For this review, take the finished solid that the model builds, in its own axes (mm). Round coordinates to 2 decimals unless told otherwise and drop trailing zeros. Order: outer loops, then holes, each group sorted by start corner. A loop starts at its lowest first (then second) coordinate and runs counter-clockwise, first axis right, second up. Notation, with made-up numbers: (8.5, -23.5) -> (60.5, -23.5) arc R26 cw to (60.5, 15.5) -> close; hole circle Ø10 at (87, 75). An arc over 180 degrees is marked (long way). Use a Markdown table: item, result. Add a question column.
1) Consider section B-B (z = -0.9). State the section outline as (x, y) points.
2) Clearance check with flat-ended pins moving along their axes: P1, Ø2, axis at x = 29.79, y = 9, coming from the -Z side; P2, Ø5.5, axis at x = 69.59, y = 23, coming from the -Z side; P3, Ø4.5, axis at x = 69.59, y = 11, coming from the -Z side. State where each tip first meets the part, or that it passes through.
3) Consider section D-D (x = 81.5). State the section outline as (y, z) points.
4) Consider section A-A (y = 28.5). State the section outline as (x, z) points, plus the area to 3 significant figures.
5) Consider section C-C (y = 16.5). State the section outline as (x, z) points, plus the area to 3 significant figures.
6) Wall thickness on line 1 along X through (y, z) = (17.75, -0.5); line 2 along X through (y, z) = (23.5, -1); line 3 along X through (y, z) = (29.5, -1.1): over which ranges is each line inside the solid? List them lowest first. Write a range as [from, to].
Autodesk Inventor part; units mm, degrees
ref_plane "YZ Plane" through (0, 0, 0) normal (1, 0, 0) x (0, 1, 0)
ref_plane "XZ Plane" through (0, 0, 0) normal (0, 1, 0) x (-1, 0, 0)
ref_plane "XY Plane" through (0, 0, 0) normal (0, 0, 1) x (1, 0, 0)
sketch "Szkic1" plane through (0, 0, 0) normal (1, 0, 0) x (0, 1, 0)
  line L0 (6, 0) -> (6, -2)
  line L1 (6, -2) -> (33, -2)
  line L2 (33, -2) -> (33, 0)
  line L3 (33, 0) -> (6, 0)
  line L4 (31, 0) -> (31, 2.3) construction
  line L5 (6, 0) -> (31, 0) construction
  line L6 (6, 5) -> (6, 0) construction
  dimension "d1" = 2
  dimension "d27" = 2
extrude "Wyciągnięcie proste1" add sketch "Szkic1" along normal blind 98
sketch "Szkic2" plane through (0, 6, -2) normal (0, 0, -1) x (-1, 0, 0)
  circle A0 centre (-69.5896, 17) radius 1.2295 construction
  circle A1 centre (-69.5896, 5) radius 1.2295 construction
  circle A2 centre (-29.7896, 3) radius 1.2295 construction
hole "Otwór1" at (69.5896, 23, -2) at (69.5896, 11, -2) at (29.7896, 9, -2) direction (0, 0, 1) diameter 3.4 depth 5.5 tip angle 118 countersink diameter 6.9 countersink angle 84.225
sketch "Szkic3" plane through (0, 6, -2) normal (0, 0, -1) x (-1, 0, 0)
  line L0 (-32.2896, 0) -> (-32.2896, 25)
  line L1 (-27.0896, 4.55) -> (-24.3896, 4.55)
  line L2 (-24.3896, 4.55) -> (-24.3896, 14.55)
  line L3 (-24.3896, 14.55) -> (-27.0896, 14.55)
  line L4 (-27.0896, 14.55) -> (-27.0896, 4.55)
  line L5 (-30.2896, 23.9) -> (-27.2896, 23.9)
  line L6 (-27.2896, 23.9) -> (-27.2896, 17.2)
  line L7 (-27.2896, 17.2) -> (-30.2896, 17.2)
  line L8 (-30.2896, 17.2) -> (-30.2896, 23.9)
  point P0 (0, -6)
  dimension "d17" = 5.2
  dimension "d18" = 4.55
  dimension "d19" = 2.7
  dimension "d20" = 10
  dimension "d21" = 2
  dimension "d22" = 17.2
  dimension "d23" = 6.7
  dimension "d24" = 3
extrude "Wyciągnięcie proste2" cut sketch "Szkic3" against normal up to next
sketch "Sketch4" plane through (0, 0, 0) normal (-1, 0, 0) x (0, 0, 1)
  line L0 (-2, 6) -> (-2, 33) construction
  line L1 (-2, 6) -> (-2, 7.1547)
  line L2 (0, 6) -> (-2, 6)
  line L3 (-2, 7.1547) -> (0, 6)
  point P0 (0, 0)
  dimension "d31" = 30
extrude "Extrusion3" cut sketch "Sketch4" against normal through all
properties part number "Tyl" material "Aluminium 6061"
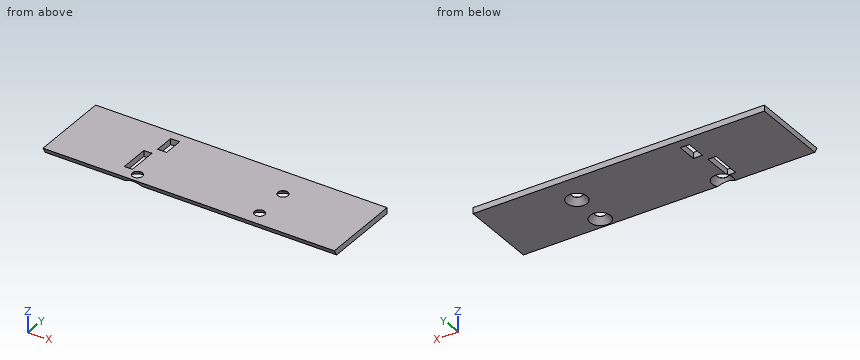
Results list:
| question | item | result |
|---|---|---|
| 1 | outline | (0, 6.52) -> (98, 6.52) -> (98, 33) -> (0, 33) -> close; hole (24.39, 10.55) -> (27.09, 10.55) -> (27.09, 20.55) -> (24.39, 20.55) -> close; hole (27.29, 23.2) -> (30.29, 23.2) -> (30.29, 29.9) -> (27.29, 29.9) -> close; hole circle Ø4.91 at (29.79, 9); hole circle Ø4.91 at (69.59, 11); hole circle Ø4.91 at (69.59, 23) |
| 2 | P1 | through |
| 2 | P2 | z = -1.23 |
| 2 | P3 | z = -0.67 |
| 3 | outline | (6, 0) -> (7.15, -2) -> (33, -2) -> (33, 0) -> close |
| 4 | outline | (0, -2) -> (27.29, -2) -> (27.29, 0) -> (0, 0) -> close; (30.29, -2) -> (98, -2) -> (98, 0) -> (30.29, 0) -> close |
| 4 | area | 190 mm2 |
| 5 | outline | (0, -2) -> (24.39, -2) -> (24.39, 0) -> (0, 0) -> close; (27.09, -2) -> (98, -2) -> (98, 0) -> (27.09, 0) -> close |
| 5 | area | 191 mm2 |
| 6 | line 1 | [0, 24.39], [27.09, 98] |
| 6 | line 2 | [0, 27.29], [30.29, 67.09], [72.09, 98] |
| 6 | line 3 | [0, 27.29], [30.29, 98] |
